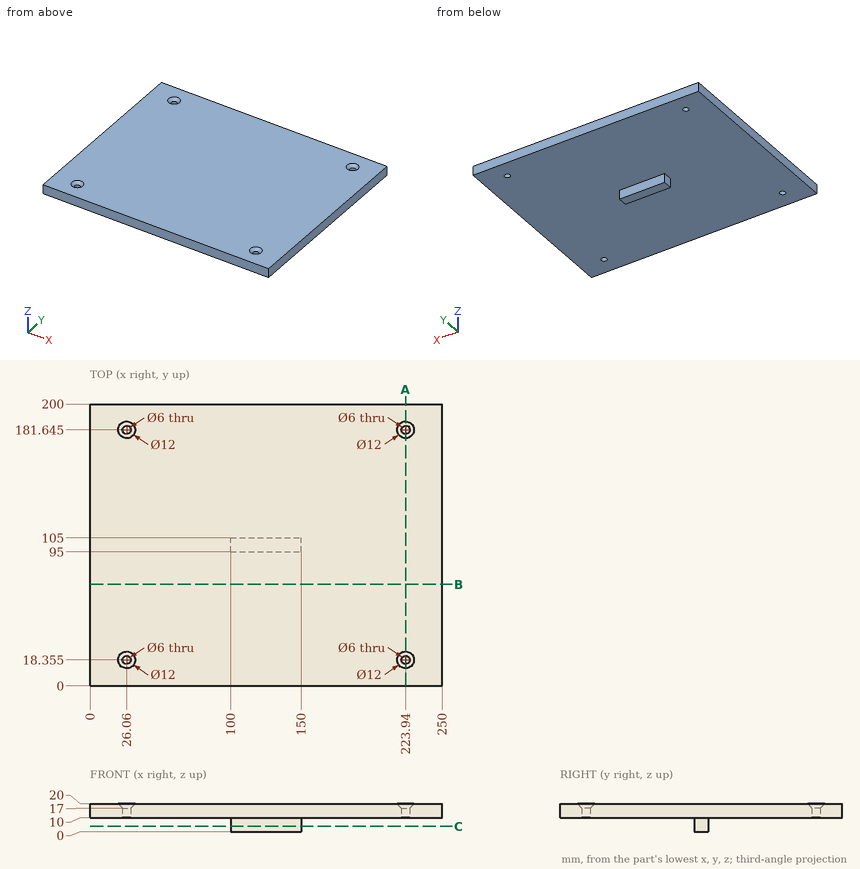
Can you work these out from the drawing? Everything is in mm from the part's minimum corner. Round coordinates to 2 decimals unless told otherwise and drop trailing zeros. Loops run counter-clockwise (first coordinate to the right, second up) from the corner with the lowest first, then second, coordinate; pieces in that order, holes last. Notation, with made-up numbers: (49.25, -20) - (82.25, -20) arc R25 cw to (82.25, 1) - close; hole circle Ø2 at (-2, 47). An arc over 180 degrees is marked (long way). Answer in a Markdown table with one row per item. Add a question column.
(1) If we section it at B-B (y = 72): Please give me the cut outline in (x, z).
(2) If we section it at A-A (x = 223.94): Please give me the cut outline in (y, z) (3 decimals), plus the area to 3 significant figures.
(3) I'm going to push flat-ended pins straight in: pin 1 (5 mm diameter, centred on y = 99, z = 5, fed in from +X); pin 2 (4 mm diameter, centred on x = 194.5, y = 104, fed in from -Z); pin 3 (4 mm diameter, centred on x = 109.5, z = 7, fed in from -Y). Where does each tip first touch, or does it pass through?
(4) If we section it at C-C (z = 4): Please give me the cut outline in (x, y).
(5) I need wall thicknesses on line 1 along Y through (x, z) = (223.94, 13.5) (3 decimals); line 2 along X through (y, z) = (17.5, 18); line 3 along Z through (x, y) = (105.5, 23.5). Which ranges of each line are inside material? Lowest first, please.
Model answer:
| question | item | result |
|---|---|---|
| 1 | outline | (0, 10) - (250, 10) - (250, 20) - (0, 20) - close |
| 2 | outline | (0, 10) - (15.355, 10) - (15.355, 17) - (12.355, 20) - (0, 20) - close; (21.355, 10) - (178.645, 10) - (178.645, 17) - (175.645, 20) - (24.355, 20) - (21.355, 17) - close; (184.645, 10) - (200, 10) - (200, 20) - (187.645, 20) - (184.645, 17) - close |
| 2 | area | 1,860 mm² |
| 3 | pin 1 | stops at x = 150 |
| 3 | pin 2 | stops at z = 10 |
| 3 | pin 3 | stops at y = 95 |
| 4 | outline | (100, 95) - (150, 95) - (150, 105) - (100, 105) - close |
| 5 | line 1 | y = 0 to 15.355, 21.355 to 178.645, 184.645 to 200 |
| 5 | line 2 | x = 0 to 22.15, 29.97 to 220.03, 227.85 to 250 |
| 5 | line 3 | z = 10 to 20 |
